from build123d import *

# Parameters (mm, degrees)
BOSS_EXTRUDE1_DEPTH       = 5
SKETCH2_W                 = 5
SKETCH2_H                 = 50
BOSS_EXTRUDE2_DEPTH       = 10
BOSS_EXTRUDE3_DEPTH       = 5
SKETCH4_R                 = 3
BOSS_EXTRUDE4_DEPTH       = 3
SKETCH5_R                 = 1.7
CUT_EXTRUDE1_DEPTH        = 3
SKETCH6_R                 = 1.65
CUT_EXTRUDE2_DEPTH        = 77.549140495
SKETCH7_R                 = 3
BOSS_EXTRUDE5_DEPTH       = 3
SKETCH8_R                 = 1.7
CUT_EXTRUDE3_DEPTH        = 3
SKETCH9_R                 = 1.65
CUT_EXTRUDE4_DEPTH        = 77.549140495
SKETCH10_W                = 23
SKETCH10_H                = 13
CUT_EXTRUDE5_DEPTH        = 77.549140495
SKETCH11_R                = 3
BOSS_EXTRUDE6_DEPTH       = 3
SKETCH12_R                = 1.7
CUT_EXTRUDE6_DEPTH        = 3
SKETCH13_R                = 1.65
CUT_EXTRUDE7_DEPTH        = 77.549140495
F_1_CLEARANCE_HOLE1_D     = 2
F_1_CLEARANCE_HOLE1_DEPTH = 25
F_4_CLEARANCE_HOLE1_D     = 3.2
FILLET1_R                 = 5
FILLET2_R                 = 5.5
FILLET3_R                 = 1.5


with BuildPart() as part:
    # Sketch1 → Boss-Extrude1 (new body)
    with BuildSketch(Plane(origin=(57.616701934, 0, 0), x_dir=(0, 0, -1), z_dir=(1, 0, 0))):
        Polygon((-6.238297922, 15), (43.761702078, 15), (33.761702078, 25), (3.761702078, 25), align=None)
    extrude(amount=-BOSS_EXTRUDE1_DEPTH)

    # Sketch2 → Boss-Extrude2 (add)
    with BuildSketch(Plane.XZ.offset(-15)):
        with Locations((55.116701934, -18.761702078)):
            Rectangle(SKETCH2_W, SKETCH2_H)
    extrude(amount=BOSS_EXTRUDE2_DEPTH)

    # Sketch3 → Boss-Extrude3 (add)
    with BuildSketch(Plane.XZ.offset(-5)):
        Polygon((5.588924157, -29.2339243), (5.588924157, -8.289479856), (20.116701934, 6.238297922), (57.616701934, 6.238297922), (57.616701934, -43.761702078), (20.116701934, -43.761702078), align=None)
    extrude(amount=BOSS_EXTRUDE3_DEPTH)

    # Sketch4 → Boss-Extrude4 (add)
    with BuildSketch(Plane(origin=(0, 5, 0), x_dir=(-1, 0, 0), z_dir=(0, 1, 0))):
        with Locations(Location((-29.616701934, -29.761702078, 0), (0, 0, 90))):
            Circle(SKETCH4_R)
    extrude(amount=BOSS_EXTRUDE4_DEPTH)

    # Sketch5 → Cut-Extrude1 (cut)
    with BuildSketch(Plane(origin=(0, 8, 0), x_dir=(-1, 0, 0), z_dir=(0, 1, 0))):
        with Locations(Location((-29.616701934, -29.761702078, 0), (0, 0, 270))):
            Circle(SKETCH5_R)
    extrude(amount=-CUT_EXTRUDE1_DEPTH, mode=Mode.SUBTRACT)

    # Sketch6 → Cut-Extrude2 (cut, through all)
    with BuildSketch(Plane.XZ):
        with Locations(Location((29.616701934, -29.761702078, 0), (0, 0, 270))):
            Circle(SKETCH6_R)
    extrude(amount=-CUT_EXTRUDE2_DEPTH, mode=Mode.SUBTRACT)

    # Sketch7 → Boss-Extrude5 (add)
    with BuildSketch(Plane(origin=(0, 5, 0), x_dir=(-1, 0, 0), z_dir=(0, 1, 0))):
        with Locations(Location((-9.616701934, -23.261702078, 0), (0, 0, 90))):
            Circle(SKETCH7_R)
    extrude(amount=BOSS_EXTRUDE5_DEPTH)

    # Sketch8 → Cut-Extrude3 (cut)
    with BuildSketch(Plane(origin=(0, 8, 0), x_dir=(-1, 0, 0), z_dir=(0, 1, 0))):
        with Locations(Location((-9.616701934, -23.261702078, 0), (0, 0, 270))):
            Circle(SKETCH8_R)
    extrude(amount=-CUT_EXTRUDE3_DEPTH, mode=Mode.SUBTRACT)

    # Sketch9 → Cut-Extrude4 (cut, through all)
    with BuildSketch(Plane.XZ):
        with Locations(Location((9.616701934, -23.261702078, 0), (0, 0, 270))):
            Circle(SKETCH9_R)
    extrude(amount=-CUT_EXTRUDE4_DEPTH, mode=Mode.SUBTRACT)

    # Sketch10 → Cut-Extrude5 (cut, through all)
    with BuildSketch(Plane.XZ):
        with Locations((34.616701934, -7.761702078)):
            Rectangle(SKETCH10_W, SKETCH10_H)
    extrude(amount=-CUT_EXTRUDE5_DEPTH, mode=Mode.SUBTRACT)

    # Sketch11 → Boss-Extrude6 (add)
    with BuildSketch(Plane(origin=(0, 5, 0), x_dir=(-1, 0, 0), z_dir=(0, 1, 0))):
        with Locations(Location((-9.616701934, -14.261702078, 0), (0, 0, 90))):
            Circle(SKETCH11_R)
    extrude(amount=BOSS_EXTRUDE6_DEPTH)

    # Sketch12 → Cut-Extrude6 (cut)
    with BuildSketch(Plane(origin=(0, 8, 0), x_dir=(-1, 0, 0), z_dir=(0, 1, 0))):
        with Locations(Location((-9.616701934, -14.261702078, 0), (0, 0, 270))):
            Circle(SKETCH12_R)
    extrude(amount=-CUT_EXTRUDE6_DEPTH, mode=Mode.SUBTRACT)

    # Sketch13 → Cut-Extrude7 (cut, through all)
    with BuildSketch(Plane.XZ):
        with Locations(Location((9.616701934, -14.261702078, 0), (0, 0, 270))):
            Circle(SKETCH13_R)
    extrude(amount=-CUT_EXTRUDE7_DEPTH, mode=Mode.SUBTRACT)

    # #1 Clearance Hole1
    with Locations(Plane(origin=(0, 0, 0), x_dir=(-1, 0, 0), z_dir=(0, -1, 0))):
        with Locations((-48.366701934, 7.761702078), (-20.866701934, 7.761702078)):
            Hole(F_1_CLEARANCE_HOLE1_D / 2, depth=F_1_CLEARANCE_HOLE1_DEPTH)

    # #4 Clearance Hole1 (through all)
    with Locations(Plane(origin=(57.616701934, 0, 0), x_dir=(0, 0, -1), z_dir=(1, 0, 0))):
        with Locations((31.461702078, 12.7), (6.061702078, 12.7)):
            Hole(F_4_CLEARANCE_HOLE1_D / 2)

    # Fillet1
    fillet1_edges = [part.edges().sort_by_distance(p)[0] for p in [
        (20.116701934, 2.5, -43.761702078),
        (20.116701934, 2.5, 6.238297922),
        (55.116701934, 25, -3.761702078),
        (55.116701934, 25, -33.761702078),
        (55.116701934, 15, -43.761702078),
        (55.116701934, 15, 6.238297922),
    ]]
    fillet(fillet1_edges, radius=FILLET1_R)

    # Fillet2
    fillet2_edges = [part.edges().sort_by_distance(p)[0] for p in [
        (5.588924157, 2.5, -29.2339243),
        (5.588924157, 2.5, -8.289479856),
    ]]
    fillet(fillet2_edges, radius=FILLET2_R)

    # Fillet3
    fillet3_edges = [part.edges().sort_by_distance(p)[0] for p in [
        (52.616701934, 25, -18.761702078),
        (52.616701934, 20, 1.238297922),
        (52.616701934, 20, -38.761702078),
        (52.616701934, 14.84234935, 5.857695585),
        (52.616701934, 24.619397663, -33.604051428),
        (52.616701934, 14.84234935, -43.38109974),
        (52.616701934, 8.964466094, -43.761702078),
        (52.616701934, 24.619397663, -3.919352728),
        (37.40223584, 5, -43.761702078),
        (12.92603635, 5, -0.952367662),
        (20.274352584, 5, 5.857695585),
        (20.274352584, 5, -43.38109974),
        (52.616701934, 8.964466094, 6.238297922),
        (5.588924157, 5, -18.761702078),
        (12.92603635, 5, -36.571036494),
        (6.007586728, 5, -29.060508585),
        (6.007586728, 5, -8.462895571),
        (37.40223584, 5, 6.238297922),
    ]]
    fillet(fillet3_edges, radius=FILLET3_R)


solid = part.part
Can you work these out from the model? Positions are in its coordinate system, mm. A direction names the side the tool comes from. Coordinates: 2 decimals unless noted, no trailing zeros. Loops run counter-clockwise (first coordinate to the right, second up) from the corner with the lowest first, then second, coordinate; pieces in that order, holes last. Notation, with made-up numbers: M 35.25,-3.75 L 44.25,-3.75 A16 cw 44.25,8.25 Z; hole C -29.75,9.5 d1. An arc over 180 degrees is marked long. Answer as CSV lines item,"result". Start each with the question number.
1. For pin 1 Ø8 at (x, z) = (19.5, 1) entering from +Y; pin 2 Ø1 at (x, z) = (10, -24) entering from +Y; pin 3 Ø4 at (y, z) = (2, -6.5) entering from -X; pin 4 Ø8 at (x, y) = (50, 22) entering from -Z, each with a flat end and sliding along its axis, tell me the tip position at first contact or that it passes through.
2. If I drill on probe 1 along X at (y, z) = (7.25, -22.5); probe 2 along Y at (x, z) = (52, -37); probe 3 along X at (y, z) = (20.75, -3), over which ranges is the centre line in solid material (lowest first)? Write a range as [from, to].
3. Suppose I cut it at A-A, the plane x = 48. List the corners of the cut face in (y, z) for me, plus the area to 3 significant figures.
4. For faces 1 (the face through (28, 8, -28)), 2 (the face through (46.117, 2, -8)), 3 (the face through (6.04, 4.57, -11.59)), which set-ups out of +Z, -Z, +X, -X, +Y, -Y let a thin tool reach every point of the face, with its end or its side?
Output:
1,pin 1,"stops at y = 5"
1,pin 2,"passes through"
1,pin 3,"stops at x = 5.99"
1,pin 4,"stops at z = -38.73"
2,probe 1,"x = [6.72, 8.1], [11.14, 12.52], [52.62, 57.62]"
2,probe 2,"y = [0, 5]"
2,probe 3,"x = [52.62, 57.62]"
3,outline,"M 0,-43.76 L 3.5,-43.76 A1.5 ccw 5,-42.26 L 5,-8.69 L 0,-8.69 Z; M 0,-6.83 L 5,-6.83 L 5,4.74 A1.5 ccw 3.5,6.24 L 0,6.24 Z"
3,area,"240 mm^2"
4,face 1,"+Z, -Z, -X, +Y"
4,face 2,"+Y, -Y"
4,face 3,"+Z, -X, +Y"
